Check sheet for the drawn part. Datum: minimum x, y, z corner. Units: mm. A direction names the side the tool comes from. Coordinates: 2 decimals unless noted, no trailing zeros. Write each question's results on one line, items separated by ' | '. Start each with the question number.
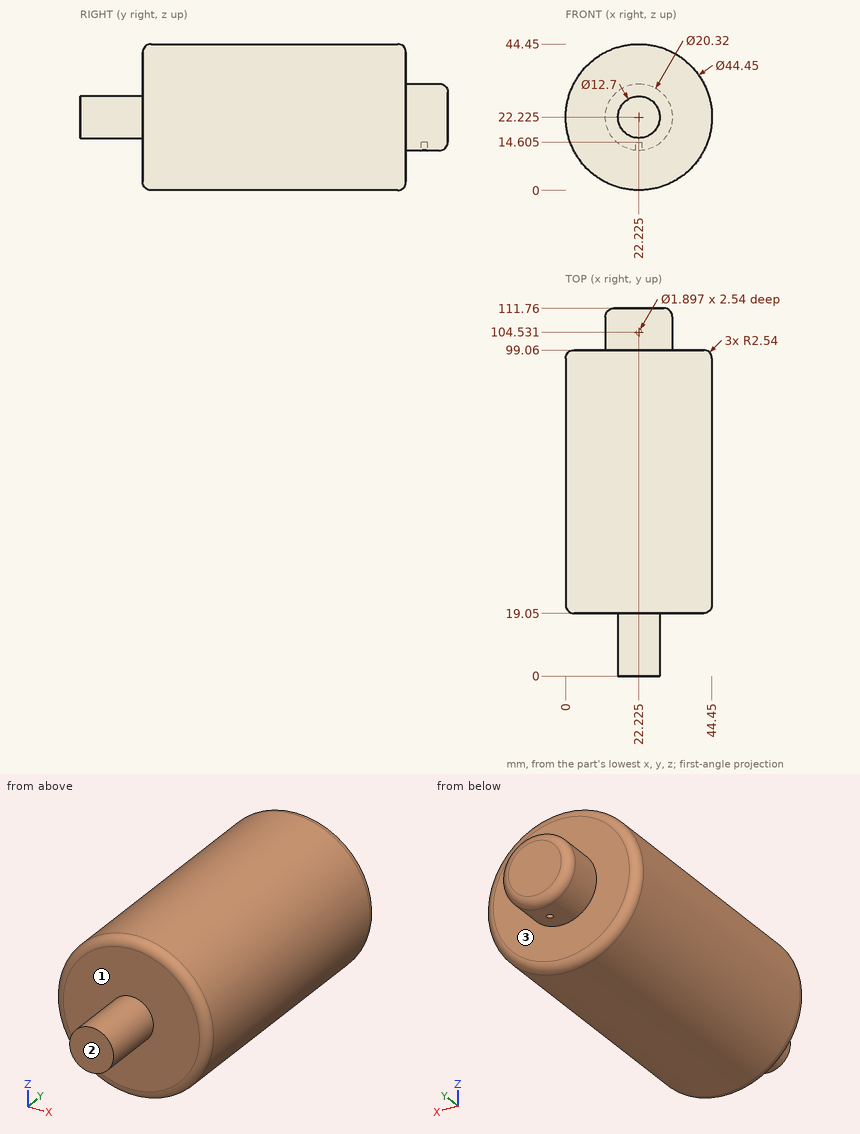
1. Tool access check on the marked faces 1, 2 and 3. Record the directions out of +Z, -Z, +X, -X, +Y, -Y that give a thin tool (end or side, any length) a straight path to the whole face; none if there is none.
2. Depth check by flat-ended pin: pin 1 Ø2 at (x, y) = (22.22, 104.53) entering from +Z (3 decimals); pin 2 Ø8 at (y, z) = (46, 29) entering from -X; pin 3 Ø4 at (y, z) = (91.5, 34) entering from -X (1 decimal). Enter the tip coordinate at first touch or a pass-through.
3. Material ranges on probe 1 along Y at (x, z) = (39, 17); probe 2 along Y at (x, z) = (21, 28.5); probe 3 along X at (y, z) = (44, 21), recorded low to high. Write a range as from..to.
Computed values:
1) face 1: -Y | face 2: +Z, -Z, +X, -X, -Y | face 3: +Y
2) pin 1: stops at z = 32.385 | pin 2: stops at x = 0.17 | pin 3: stops at x = 2.3
3) probe 1: y = 19.05..99.06 | probe 2: y = 19.05..111.76 | probe 3: x = 0.03..44.42
